Geometry: final body of the model. Coordinates: model frame, mm. A direction names the side the tool comes from. Give positions to 0.01 mm unless a question says otherwise; leave off trailing zeros. Write each loop counter-clockwise with the first axis right and the second up, starting at its lowest first coordinate (ties: lowest second). Pieces come first, ordered by that corner, then holes.
from build123d import *

# Parameters (mm, degrees)
F0_W           = 100
F0_H           = 63
F1_DEPTH       = 12
F2_R           = 25
F3_R           = 6
F4_DEPTH       = 12
F5_R           = 6
F6_DEPTH       = 12
F7_R           = 25
F7_R_2         = 12.5
F8_DEPTH       = 44
F12_DEPTH      = 10
F14_DEPTH      = 10
F16_W          = 27
F16_H          = 32
F17_DEPTH      = 23
F18_W          = 10
F18_H          = 34
F21_DEPTH      = 10
F22_W          = 3
F22_H          = 60
F23_DEPTH      = 25
F23_DEPTH_BACK = 25
F24_R          = 6
F25_DEPTH      = 63.501


# Not quite as in the source:
# - a feature of the source that left no trace in its solid (it failed there, or was rolled back) is left out


with BuildPart() as f1:
    # F0 (on Top) → F1 (new body)
    with BuildSketch(Plane.XY):
        Rectangle(F0_W, F0_H)
    extrude(amount=F1_DEPTH)

    # F2
    f2_edges = [f1.edges().sort_by_distance(p)[0] for p in [
        (-50, -31.5, 6),
        (50, -31.5, 6),
    ]]
    fillet(f2_edges, radius=F2_R)

    # F3 (on face) → F4 (cut, through all)
    with BuildSketch(Plane.XY.offset(12)):
        with Locations((-25, -6.5)):
            Circle(F3_R)
    extrude(amount=-F4_DEPTH, mode=Mode.SUBTRACT)

    # F5 (on face) → F6 (cut, through all)
    with BuildSketch(Plane.XY.offset(12)):
        with Locations((25, -6.5)):
            Circle(F5_R)
    extrude(amount=-F6_DEPTH, mode=Mode.SUBTRACT)



with BuildPart() as f8:
    # F7 (on face) → F8 (new body)
    with BuildSketch(Plane(origin=(0, 31.5, 0), x_dir=(-1, 0, 0), z_dir=(0, 1, 0))):
        with Locations((0, 100)):
            Circle(F7_R)
        with Locations((0, 100)):
            Circle(F7_R_2, mode=Mode.SUBTRACT)
    extrude(amount=-F8_DEPTH)


with BuildPart() as f1_1:
    add(f1.part)

    add(f8.part)  # F12 merges F8
    # F11 (on face) → F12 (join)
    with BuildSketch(Plane(origin=(0, 31.5, 0), x_dir=(-1, 0, 0), z_dir=(0, 1, 0))):
        Polygon((-25, 100), (-50, 12), (-25, 12), align=None)
    extrude(amount=-F12_DEPTH)

    # F13 (on face) → F14 (join)
    with BuildSketch(Plane(origin=(0, 31.5, 0), x_dir=(-1, 0, 0), z_dir=(0, 1, 0))):
        Polygon((25, 100), (25, 12), (50, 12), align=None)
        with BuildLine():
            Line((-25, 12), (25, 12))
            Line((25, 12), (25, 100))
            ThreePointArc((25, 100), (0, 75), (-25, 100))
            Line((-25, 100), (-25, 12))
        make_face()
    extrude(amount=-F14_DEPTH)

    # F16 (on offset) → F17 (join)
    with BuildSketch(Plane.XY.offset(120)):
        with Locations((0, 9.5)):
            Rectangle(F16_W, F16_H)
    extrude(amount=F17_DEPTH)

    # F18 (on face) → F19 (join, up to the next surface of F1)
    with BuildSketch(Plane.XY.offset(12)):
        with Locations((0, 4.5)):
            Rectangle(F18_W, F18_H)
    extrude(until=Until.NEXT)

    # F20 (on face) → F21 (join)
    with BuildSketch(Plane(origin=(-5, 0, 0), x_dir=(0, -1, 0), z_dir=(-1, 0, 0))):
        Polygon((31.4197465777, 12), (12.5, 75.5051025722), (12.5, 12), align=None)
    extrude(amount=-F21_DEPTH)

    # F22 (on offset) → F23 (cut, two sides)
    with BuildSketch(Plane.XY.offset(120)) as f23_sk:
        with Locations((0, 3.3281182433)):
            Rectangle(F22_W, F22_H)
    extrude(amount=-F23_DEPTH, mode=Mode.SUBTRACT)
    extrude(f23_sk.sketch, amount=F23_DEPTH_BACK, mode=Mode.SUBTRACT)

    # F24 (on face) → F25 (cut, through all)
    with BuildSketch(Plane.YZ.offset(13.5)):
        with Locations((9.5, 131)):
            Circle(F24_R)
    extrude(amount=-F25_DEPTH, mode=Mode.SUBTRACT)


solid = f1_1.part
Q1. Access query for faces 4 (the flat face through (23, 21.5, 47)), 5 (the flat face through (-22, 21.5, 47)), 6 (the flat face through (-1.5, 9.2, 124.5)). Directions: +Z, -Z, +X, -X, +Y, -Y. A direction counts if a zero-diameter tool reaches every point of the face in a straight line with its end or side. Return the directions, or none.
Filled sheet:
face 4: +X, -Y
face 5: -X, -Y
face 6: +Z, +Y, -Y
Q2. Ray query, line 1 along X through (y, z) = (-6, 3); line 2 along Z through (x, y) = (10, 9); line 3 along Y through (x, z) = (21, 69.5). Return the intervals inside material, ascending.
Filled sheet:
line 1: x = -50 to -30.98, -19.02 to 19.02, 30.98 to 50
line 2: z = 0 to 12, 77.09 to 92.5, 107.5 to 125.02, 136.98 to 143
line 3: y = 21.5 to 31.5
Q3. Pin query (flat end, axial travel): P1, Ø22.5, axis at x = -23, z = 73, coming from the -Y side; P2, Ø12, axis at x = 14.5, y = -14.5, coming from the +Z side; P3, Ø13.5, axis at x = 27, z = 64.5, coming from the -Y side. Return the tip coordinate at first contact, or that it passes through.
Filled sheet:
P1: stops at y = -12.5
P2: stops at z = 123.38
P3: stops at y = 21.5
Q4. Section B-B on z = 131. Output: boundary loops of the cut face in (x, y).
Filled sheet:
outline: (-13.5, -6.5) - (-1.5, -6.5) - (-1.5, 3.5) - (-13.5, 3.5) - close; (-13.5, 15.5) - (-1.5, 15.5) - (-1.5, 25.5) - (-13.5, 25.5) - close; (1.5, -6.5) - (13.5, -6.5) - (13.5, 3.5) - (1.5, 3.5) - close; (1.5, 15.5) - (13.5, 15.5) - (13.5, 25.5) - (1.5, 25.5) - close
Q5. Section D-D on x = 40.5. Output: boundary loops of the cut face in (y, z), plus the area to 3 significant figures.
Filled sheet:
outline: (-26.12, 0) - (31.5, 0) - (31.5, 45.44) - (21.5, 45.44) - (21.5, 12) - (-26.12, 12) - close
area: 1,030 mm2
Q6. Pull-direction query (Z, two-part tool) for faces 1 (the flat face through (5, 1, 44)), 2 (the flat face through (-37.675, 26.57, 55.384)), 3 (the flat face through (-8, 25.5, 134)); classes: released by +Z, released by -Z, zero draft, split by the parting line, or undercut.
Filled sheet:
face 1: undercut
face 2: released by +Z
face 3: zero draft
Q7. Section C-C on z = 21.5. Output: boundary loops of the cut face in (x, y).
Filled sheet:
outline: (-47.3, 21.5) - (-5, 21.5) - (-5, -28.59) - (5, -28.59) - (5, 21.5) - (47.3, 21.5) - (47.3, 31.5) - (-47.3, 31.5) - close
Q8. Section A-A on y = 9.5. Output: boundary loops of the cut face in (x, z).
Filled sheet:
outline: (-50, 0) - (50, 0) - (50, 12) - (5, 12) - (5, 75.51) arc R25 ccw to (13.5, 121.04) - (13.5, 125) - (1.5, 125) - (1.5, 112.41) arc R12.5 cw (long way) to (-1.5, 112.41) - (-1.5, 125) - (-13.5, 125) - (-13.5, 121.04) arc R25 ccw to (-5, 75.51) - (-5, 12) - (-50, 12) - close; (-13.5, 137) - (-1.5, 137) - (-1.5, 143) - (-13.5, 143) - close; (1.5, 137) - (13.5, 137) - (13.5, 143) - (1.5, 143) - close
